Verification items for the finished model (mm, model axes). A direction names the side the tool comes from. Round coordinates to 2 decimals unless told otherwise and drop trailing zeros. Write each loop counter-clockwise with the first axis right and the second up, starting at its lowest first coordinate (ties: lowest second). Pieces come first, ordered by that corner, then holes. Notation, with made-up numbers: (-31.5, -35) - (4.5, -35) arc R20 cw to (4.5, -19) - close; hole circle Ø1 at (-7, 5). An arc over 180 degrees is marked (long way). Answer as a JSON object with one key per item and string values. Group by question number.
1) Section check A-A (x = 0). Enter the section's corners in (y, z).
2) Thickness scan on line 1 (Z direction, x = -3.5, y = 1); line 2 (Y direction, x = 0, z = -0.8); line 3 (Y direction, x = 0, z = -1.95). Record the ranges inside material, lowest first.
3) Set-up check for faces 1 (the flat face through (1.682, 7, 7)), 2 (the flat face through (5, 0, 7.5)), 3 (the flat face through (3, -11, 0)): record each of +Z, -Z, +X, -X, +Y, -Y from which the full face is reachable in a straight line by a thin tool's end or side.
4) Section check C-C (z = -2). Enter the section's corners in (x, y), then the cut area to 3 significant figures.
5) Section check B-B (z = 2.75). Enter the section's corners in (x, y), then the cut area to 3 significant figures.
6) Go/stop test with flat-tipped pins: pin 1 Ø1.4 at (y, z) = (4.5, 7) entering from -X; pin 2 Ø2 at (y, z) = (6, -1) entering from +X; pin 3 Ø4 at (x, y) = (-3.5, 11) entering from +Z; pin 4 Ø3.5 at (x, y) = (0, 0) entering from +Z. Record where each tip stops, or that it passes through.
Autodesk Fusion 360 part; units mm, degrees
sketch "Sketch1" plane through (0, 0, 0) normal (0, 0, 1) x (1, 0, 0)
  circle A0 centre (0, 0) radius 11
  circle A1 centre (0, 0) radius 2.85
  dimension "d1" = 22
  dimension "d2" = 5.7
extrude "Extrude1" add sketch "Sketch1" along normal blind 7.5
sketch "Sketch2" plane through (0, 0, 7.5) normal (0, 0, 1) x (-1, 0, 0)
  circle A0 centre (0, 0) radius 2.85
  circle A1 centre (0, 0) radius 11
  line L0 (-1.6821, -10.8706) -> (-1.6821, 10.8706)
extrude "Extrude2" cut sketch "Sketch2" against normal blind 1.7 contours A0 A1 L0 picked at (-0.6386, 8.2391)
sketch "Sketch3" plane through (0, 0, 0) normal (0, 0, -1) x (1, 0, 0)
  circle A0 centre (0, 0) radius 2.85
  circle A1 centre (0, 0) radius 11
  circle A2 centre (0, 0) radius 14
  dimension "d7" = 28
extrude "Extrude3" add sketch "Sketch3" against normal blind 3.4 draft 30 from surface at 3.4 contours A1 | A2
extrude "Extrude4" cut sketch "Sketch2" against normal up to surface (10.9 mm away) contours A0 L0 | A0 L0
Returned:
{
 "1": {"outline": "(-15.96, 0) - (-14, -3.4) - (-2.85, -3.4) - (-2.85, 5.8) - (-11, 5.8) - (-11, 0) - close; (2.85, -3.4) - (14, -3.4) - (15.96, 0) - (11, 0) - (11, 5.8) - (2.85, 5.8) - close"},
 "2": {"line 1": "-3.4 to 5.8", "line 2": "-15.5 to -2.85, 2.85 to 15.5", "line 3": "-14.84 to -2.85, 2.85 to 14.84"},
 "3": {"face 1": "+Z, -X, +Y, -Y", "face 2": "+Z, +X, -X, +Y, -Y", "face 3": "+Z"},
 "4": {"outline": "circle Ø29.62 at (0, 0); hole circle Ø5.7 at (0, 0)", "area": "663 mm2"},
 "5": {"outline": "circle Ø22 at (0, 0); hole circle Ø5.7 at (0, 0)", "area": "355 mm2"},
 "6": {"pin 1": "x = 1.68", "pin 2": "x = 14.9", "pin 3": "z = 5.8", "pin 4": "through"}
}
